Geometry: final body of the model. Coordinates: model frame, mm. A direction names the side the tool comes from. Coordinates: 2 decimals unless noted, no trailing zeros. Write each loop counter-clockwise with the first axis right and the second up, starting at its lowest first coordinate (ties: lowest second). Pieces come first, ordered by that corner, then holes. Notation, with made-up numbers: (47, 27) -> (83, 27) arc R22 cw to (83, 58) -> close; hole circle Ø7 at (4, 19.25). An arc over 180 degrees is marked (long way). One line per item, written item: value.
```python
from build123d import *

# Parameters (mm, degrees)
SKETCH1_W                  = 45
SKETCH1_H                  = 1.2
BOSS_EXTRUDE1_DEPTH        = 25
SKETCH2_W                  = 42.4
SKETCH2_H                  = 22.4
SKETCH2_W_2                = 40.4
SKETCH2_H_2                = 20.4
EXTRUDE_THIN1_DEPTH        = 1.5
F_6_0_204_DIAMETER_HOLE1_D = 3.9
SKETCH6_W                  = 41
SKETCH6_H                  = 21
SKETCH6_W_2                = 38.6
SKETCH6_H_2                = 18.6
EXTRUDE_THIN2_DEPTH        = 2.5
FILLET1_R                  = 0.5


with BuildPart() as part:
    # Sketch1 → Boss-Extrude1 (new body)
    with BuildSketch(Plane.XY):
        with Locations((22.5, 0.6)):
            Rectangle(SKETCH1_W, SKETCH1_H)
    extrude(amount=-BOSS_EXTRUDE1_DEPTH)

    # Sketch2 → Extrude-Thin1 (add)
    with BuildSketch(Plane(origin=(0, 1.2, 0), x_dir=(1, 0, 0), z_dir=(0, 1, 0))):
        with Locations((22.5, 12.5)):
            Rectangle(SKETCH2_W, SKETCH2_H)
        with Locations((22.5, 12.5)):
            Rectangle(SKETCH2_W_2, SKETCH2_H_2, mode=Mode.SUBTRACT)
    extrude(amount=EXTRUDE_THIN1_DEPTH)

    # #6 (0.204) Diameter Hole1 (through all)
    with Locations(Plane(origin=(0, 0, 0), x_dir=(-1, 0, 0), z_dir=(0, -1, 0))):
        with Locations((-5, 12.5), (-40, 12.5)):
            Hole(F_6_0_204_DIAMETER_HOLE1_D / 2)

    # Sketch6 → Extrude-Thin2 (add)
    with BuildSketch(Plane(origin=(0, 1.2, 0), x_dir=(1, 0, 0), z_dir=(0, 1, 0))):
        with Locations((22.5, 12.5)):
            Rectangle(SKETCH6_W, SKETCH6_H)
        with Locations((22.5, 12.5)):
            Rectangle(SKETCH6_W_2, SKETCH6_H_2, mode=Mode.SUBTRACT)
    extrude(amount=EXTRUDE_THIN2_DEPTH)

    # Fillet1
    fillet1_edges = [part.edges().sort_by_distance(p)[0] for p in [
        (38.05, 0, -12.5),
        (3.05, 0, -12.5),
        (22.5, 0, 0),
        (45, 0, -12.5),
        (0, 0, -12.5),
        (22.5, 0, -25),
    ]]
    fillet(fillet1_edges, radius=FILLET1_R)


solid = part.part
```
(1) First-contact query: pin 1 (8 mm diameter, centred on x = 26, z = -11.5, fed in from -Y); pin 2 (1 mm diameter, centred on y = 2, z = -19, fed in from -X); pin 3 (3.5 mm diameter, centred on x = 5, z = -12.5, fed in from -Y); pin 4 (0.8 mm diameter, centred on y = 2, z = -16, fed in from +X). Flat tips, straight axial feed; report the tip coordinate or a pass-through.
Responses:
pin 1: stops at y = 0
pin 2: stops at x = 1.3
pin 3: passes through
pin 4: stops at x = 43.7
(2) Section C-C (y = 2). Return the cut outline in (x, z), then the cut area to 3 significant figures.
Responses:
outline: (1.3, -23.7) -> (43.7, -23.7) -> (43.7, -1.3) -> (1.3, -1.3) -> close; hole (3.2, -21.8) -> (41.8, -21.8) -> (41.8, -3.2) -> (3.2, -3.2) -> close
area: 232 mm2
(3) Line query: line 1 (X direction, y = 1.05, z = -12.5); line 2 (X direction, y = 1.8, z = -10.5); line 3 (Z direction, x = 40, y = 0.65). Output: solid intervals per line, ascending. Write a range as [from, to].
Responses:
line 1: x = [0, 3.05], [6.95, 38.05], [41.95, 45]
line 2: x = [1.3, 3.2], [41.8, 43.7]
line 3: z = [-25, -14.45], [-10.55, 0]
(4) Section A-A (x = 40). Return the cut outline in (y, z).
Responses:
outline: (0, -24.5) arc R0.5 ccw to (0.5, -25) -> (1.2, -25) -> (1.2, -23.7) -> (2.7, -23.7) -> (2.7, -23) -> (3.7, -23) -> (3.7, -21.8) -> (1.2, -21.8) -> (1.2, -14.45) -> (0.5, -14.45) arc R0.5 ccw to (0, -14.95) -> close; (0, -10.05) arc R0.5 ccw to (0.5, -10.55) -> (1.2, -10.55) -> (1.2, -3.2) -> (3.7, -3.2) -> (3.7, -2) -> (2.7, -2) -> (2.7, -1.3) -> (1.2, -1.3) -> (1.2, 0) -> (0.5, 0) arc R0.5 ccw to (0, -0.5) -> close
(5) Section D-D (z = -15.5). Return the cut outline in (x, y), then the cut area to 3 significant figures.
Responses:
outline: (0, 0.5) arc R0.5 ccw to (0.5, 0) -> (44.5, 0) arc R0.5 ccw to (45, 0.5) -> (45, 1.2) -> (43.7, 1.2) -> (43.7, 2.7) -> (43, 2.7) -> (43, 3.7) -> (41.8, 3.7) -> (41.8, 1.2) -> (3.2, 1.2) -> (3.2, 3.7) -> (2, 3.7) -> (2, 2.7) -> (1.3, 2.7) -> (1.3, 1.2) -> (0, 1.2) -> close
area: 62.0 mm2
(6) Pull-direction query (X, two-part tool) for faces 1 (the flat face through (22, 2, -3.2)), 2 (the flat face through (2, 3, -12)), 3 (the flat face through (22, 2, -23.7)); classes: released by +X, released by -X, zero draft, split by the parting line, or undercut.
Responses:
face 1: undercut
face 2: released by -X
face 3: zero draft
(7) Reachability of faces 4 (the flat face through (43.7, 2, -12)), 5 (the flat face through (22, 3, -23)), 6 (the flat face through (41.8, 2, -12)) from +Z, -Z, +X, -X, +Y, -Y: full face, straight path, thin tool, end or side. Return the list, or none.
Responses:
face 4: +Z, -Z, +X, +Y
face 5: -Z, +X, -X, +Y
face 6: +Y
(8) Section B-B (z = -12.5). State how many separate pieces and enclosed holes the cut face has, then the cut area to 3 significant figures.
Responses:
separate pieces: 3
enclosed holes: 0
area: 52.4 mm2
